The listing builds one solid part. Answer for the finished solid, in the listing's coordinates (mm). A direction names the side the tool comes from. Give positions to 0.01 mm unless a question says otherwise; leave off trailing zeros. Loops run counter-clockwise (first coordinate to the right, second up) from the corner with the lowest first, then second, coordinate; pieces in that order, holes last.
Item 1: A tool of negligible diameter and unlimited length cuts with its end or side. For faces 4 (the face through (3, 0, 49.85)), 5 (the face through (-5, 0, 44.85)), 6 (the face through (-4, 4, 35)), from which of +Z, -Z, +X, -X, +Y, -Y can it reach the whole face along a straight path? Write none if from no direction.
Item 2: Section C-C, the plane z = 29 is taken. Give the vertices of the cut face in (x, y).
Item 3: The mould has two halves that part along Y. Classify faces 1 (the face through (2.44, 0.54, 45.79)), 2 (the face through (0, 0, 0)), 3 (the face through (5.54, 2.3, 42.32)): pulls with the +Y half, pulls with the -Y half, needs draft (parallel to the pull), parting line crosses it, or undercut.
Item 4: Each of these flat-tipped pins is pushed along its axis until it touches: pin 1 Ø5.5 at (y, z) = (-2, 48) entering from -X; pin 2 Ø2 at (x, z) = (-2.5, 36.5) entering from -Y; pin 3 Ø1 at (y, z) = (-1, 43) entering from +X. Where does it stop, or does it pass through?
Item 5: Consider line 1 along Y through (x, z) = (0, 44); line 2 along X through (y, z) = (0, 47.25). Determine where each line is inside the solid, lowest interval first.
Item 6: Section B-B, the plane z = 35.5 is taken. Give the vertices of the cut face in (x, y), and give its area (3 significant figures).
Item 7: Section A-A, the plane x = -3.25 is taken. Give the vertices of the cut face in (y, z).
Autodesk Inventor part; units mm, degrees
ref_plane "作業平面1" through (0, 6, 49.85) normal (0, 1, 0) x (-1, 0, 0)
ref_plane "YZ Plane" through (0, 0, 0) normal (1, 0, 0) x (0, 1, 0)
ref_plane "XZ Plane" through (0, 0, 0) normal (0, 1, 0) x (-1, 0, 0)
sketch "スケッチ1" plane through (0, 0, 0) normal (0, 0, 1) x (1, 0, 0)
  point P0 (0, 0)
sketch "スケッチ2" plane through (0, 0, 0) normal (0, 0, 1) x (1, 0, 0)
  circle A0 centre (0, 0) radius 5
  dimension "d0" = 10
extrude "押し出し1" add sketch "スケッチ2" along normal blind 35
thread "ねじ1"
sketch "スケッチ3" plane through (0, 0, 35) normal (0, 0, 1) x (1, 0, 0)
  point P0 (0, 0)
sketch "スケッチ4" plane through (0, 0, 35) normal (0, 0, 1) x (1, 0, 0)
  circle A0 centre (0, 0) radius 6
  dimension "d5" = 12
extrude "押し出し2" add sketch "スケッチ4" along normal blind 14.85
sketch "スケッチ5" plane through (0, 0, 49.85) normal (0, 0, 1) x (1, 0, 0)
  line L0 (0, 0) -> (0, 6)
  circle A0 centre (0, 0) radius 6
ref_plane "作業平面1" through (0, 6, 49.85) normal (0, 1, 0) x (-1, 0, 0)
sketch "スケッチ9" plane through (0, 0, 49.85) normal (0, 0, 1) x (1, 0, 0)
  point P0 (0, 0)
  point P1 (0, 0)
hole "穴2" at (0, 0, 49.85) direction (0, 0, -1) diameter 5 depth 8 tip angle 118
thread "ねじ3"
sketch "スケッチ10" plane through (0, 0, 49.85) normal (0, 0, 1) x (1, 0, 0)
  arc A0 (-4, 4.4721) -> (-4, -4.4721) centre (0, 0) ccw
  line L0 (-4, 0) -> (-4, 4.4721)
  line L1 (-4, 0) -> (-4, -4.4721)
  dimension "d34" = 12
  dimension "d35" = 4
extrude "押し出し4" cut sketch "スケッチ10" against normal blind 5
properties part number "回転アーム付き計測輪シャフト"
Worked answers:
1. face 4: +Z, +X, -X, +Y, -Y
1. face 5: +Z, -X, +Y, -Y
1. face 6: -Z
2. outline: circle Ø10 at (0, 0)
3. face 1: undercut
3. face 2: needs draft
3. face 3: parting line crosses it
4. pin 1: stops at x = -4
4. pin 2: stops at y = -5.81
4. pin 3: stops at x = 5.98
5. line 1: y = -6 to -2.5, 2.5 to 6
5. line 2: x = -4 to -2.5, 2.5 to 6
6. outline: circle Ø12 at (0, 0)
6. area: 113 mm2
7. outline: (-5.04, 35) - (-3.8, 35) - (-3.8, 0) - (3.8, 0) - (3.8, 35) - (5.04, 35) - (5.04, 49.85) - (-5.04, 49.85) - close
